Geometry: final body of the model. Coordinates: model frame, mm. Face numbers are marked on the shaded views. A direction names the side the tool comes from. Give positions to 0.01 mm unless a question says otherwise; leave off trailing zeros. Loops run counter-clockwise (first coordinate to the right, second up) from the corner with the lowest first, then second, coordinate; pieces in that order, holes last.
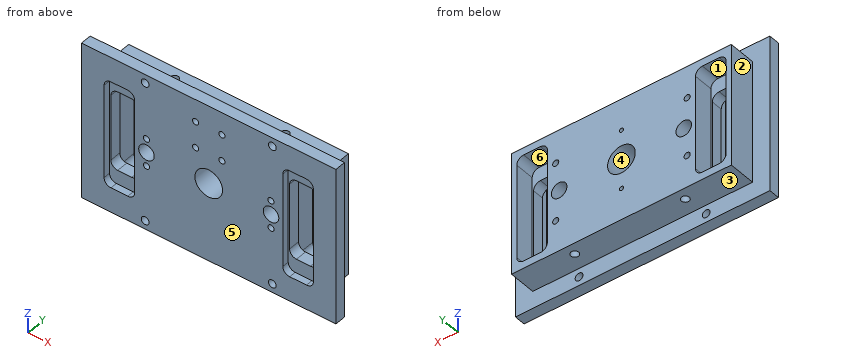
```python
from build123d import *

# Parameters (mm, degrees)
MAIN_SKETCH_W                         = 73.5
MAIN_SKETCH_H                         = 45.5
MAIN_SKETCH_W_2                       = 8.85
MAIN_SKETCH_H_2                       = 31.2
MAIN_SKETCH_R                         = 2.2479
LIP_DEPTH                             = 3.175
MOUNTING_BASE_OUTLINE_W               = 63.5
MOUNTING_BASE_OUTLINE_H               = 35.5
MOUNTING_BASE_OUTLINE_R               = 2.2479
MOUNTING_BASE_OUTLINE_R_2             = 4
MOUNTING_BASE_DEPTH                   = 11
HEATER_CART_4_40_TAPS_D               = 2.2606
HEATER_CART_4_40_TAPS_DEPTH           = 8.255
HEATER_CART_4_40_TAPS_TIP             = 0.679152758
HEATER_CART_4_40_TAPS_ON_FACE_2_D     = 2.2606
HEATER_CART_4_40_TAPS_ON_FACE_2_DEPTH = 8.255
HEATER_CART_4_40_TAPS_ON_FACE_2_TIP   = 0.679152758
MAIN_SKETCH_12_W                      = 8.85
MAIN_SKETCH_12_H                      = 31.2
MAIN_SKETCH_12_R                      = 0.285
BOTTOM_SQUARE_CUTOUT_DEPTH            = 2
SQUARE_MICRO_D_CUTOUT_START           = 5.3
SQUARE_MICRO_D_CUTOUT_OUTLINE_W       = 8.85
SQUARE_MICRO_D_CUTOUT_OUTLINE_H       = 31.2
SQUARE_MICRO_D_CUTOUT_OUTLINE_R       = 0.285
SQUARE_MICRO_D_CUTOUT_DEPTH           = 5.7
SKETCH15_W                            = 8.067488146
SKETCH15_H                            = 23.070933647
CUT_EXTRUDE1_DEPTH                    = 11
INTERNAL_CORNER_CUTOUTS_FILLET_R      = 2
CHIP_CLAMP_0_80_TAPS_AT_2_COUNT       = 2
CHIP_CLAMP_0_80_TAPS_AT_2_PITCH       = 17.1232
CHIP_CLAMP_0_80_TAPS_AT_3_COUNT       = 2
CHIP_CLAMP_0_80_TAPS_AT_3_PITCH       = 17.1232
F_2_56_CLOSE_CLEAR_43_0_089_D         = 2.2606
PCB_2_56_TAPS_D                       = 1.778
PCB_2_56_TAPS_DEPTH                   = 5.734
PCB_2_56_TAPS_TIP                     = 0.53416509
BOTTOM_COVER_2_56_TAPS_D              = 1.778
BOTTOM_COVER_2_56_TAPS_DEPTH          = 5.734
BOTTOM_COVER_2_56_TAPS_TIP            = 0.53416509
F_2_56_TAPPED_HOLE1_D                 = 1.778
F_2_56_TAPPED_HOLE1_DEPTH             = 5.734
F_2_56_TAPPED_HOLE1_TIP               = 0.53416509


# Read off the part's stored shape, not the designer's step: Mounting_Base, Square_Micro_D_Cutout
with BuildPart() as part:
    # Main_Sketch → Lip (new body)
    with BuildSketch(Plane(origin=(0, 0, 0), x_dir=(1, 0, 0), z_dir=(0, 1, 0))):
        with Locations((36.75, -22.75)):
            Rectangle(MAIN_SKETCH_W, MAIN_SKETCH_H)
        with Locations((10.925, -22.749999985)):
            Rectangle(MAIN_SKETCH_W_2, MAIN_SKETCH_H_2, mode=Mode.SUBTRACT)
        with Locations(Location((18.75, -22.75, 0), (0, 0, 270))):
            Circle(MAIN_SKETCH_R, mode=Mode.SUBTRACT)
        with BuildLine():
            ThreePointArc((31.675, -20.175), (29.907233047, -15.907233047), (34.175, -17.675))
            Line((34.175, -17.675), (39.325, -17.675))
            ThreePointArc((39.325, -17.675), (43.592766953, -15.907233047), (41.825, -20.175))
            Line((41.825, -20.175), (41.825, -25.325))
            ThreePointArc((41.825, -25.325), (43.592766953, -29.592766953), (39.325, -27.825))
            Line((39.325, -27.825), (34.175, -27.825))
            ThreePointArc((34.175, -27.825), (29.907233047, -29.592766953), (31.675, -25.325))
            Line((31.675, -25.325), (31.675, -20.175))
        make_face(mode=Mode.SUBTRACT)
        with Locations(Location((54.75, -22.75, 0), (0, 0, 270))):
            Circle(MAIN_SKETCH_R, mode=Mode.SUBTRACT)
    extrude(amount=LIP_DEPTH)

    # Mounting_Base outline → Mounting_Base (add)
    with BuildSketch(Plane(origin=(0, 0, 0), x_dir=(1, 0, 0), z_dir=(0, 1, 0))):
        with Locations((36.75, -22.75)):
            Rectangle(MOUNTING_BASE_OUTLINE_W, MOUNTING_BASE_OUTLINE_H)
        with Locations((18.75, -22.75)):
            Circle(MOUNTING_BASE_OUTLINE_R, mode=Mode.SUBTRACT)
        with Locations((54.75, -22.75)):
            Circle(MOUNTING_BASE_OUTLINE_R, mode=Mode.SUBTRACT)
        with Locations((36.75, -22.75)):
            Circle(MOUNTING_BASE_OUTLINE_R_2, mode=Mode.SUBTRACT)
    extrude(amount=MOUNTING_BASE_DEPTH)

    # Heater_Cart_#4-40_Taps
    with Locations(Plane(origin=(52.725, 7.825, 5), x_dir=(-1, 0, 0), z_dir=(0, 0, -1))):
        with Locations((0, 0), (31.95, 0)):
            Hole(HEATER_CART_4_40_TAPS_D / 2, depth=HEATER_CART_4_40_TAPS_DEPTH)
            with Locations((0, 0, -(HEATER_CART_4_40_TAPS_DEPTH + HEATER_CART_4_40_TAPS_TIP / 2))):  # 118° drill point
                Cone(0, HEATER_CART_4_40_TAPS_D / 2, HEATER_CART_4_40_TAPS_TIP, mode=Mode.SUBTRACT)

    # Heater_Cart_#4-40_Taps on face 2
    with Locations(Plane(origin=(20.775, 7.825, 40.5), x_dir=(1, 0, 0), z_dir=(0, 0, 1))):
        with Locations((0, 0), (31.95, 0)):
            Hole(HEATER_CART_4_40_TAPS_ON_FACE_2_D / 2, depth=HEATER_CART_4_40_TAPS_ON_FACE_2_DEPTH)
            with Locations((0, 0, -(HEATER_CART_4_40_TAPS_ON_FACE_2_DEPTH + HEATER_CART_4_40_TAPS_ON_FACE_2_TIP / 2))):  # 118° drill point
                Cone(0, HEATER_CART_4_40_TAPS_ON_FACE_2_D / 2, HEATER_CART_4_40_TAPS_ON_FACE_2_TIP, mode=Mode.SUBTRACT)

    # Main_Sketch<12> → Bottom_square_cutout (cut)
    # profile 1 of 2: a face of its own
    with BuildSketch(Plane(origin=(0, 0, 0), x_dir=(1, 0, 0), z_dir=(0, 1, 0))):
        with Locations((10.925, -22.749999985)):
            Rectangle(MAIN_SKETCH_12_W, MAIN_SKETCH_12_H)
        with BuildLine():
            ThreePointArc((10.385689992, -35.285466808), (9.155254643, -35.471894814), (7.986136174, -35.045410869))
            ThreePointArc((7.986136174, -35.045410869), (7.18175843, -34.143309058), (6.891255927, -32.970099985))
            Line((6.891255927, -32.970099985), (6.891255927, -12.529899985))
            ThreePointArc((6.891255927, -12.529899985), (7.18175845, -11.356690961), (7.986136174, -10.454589189))
            ThreePointArc((7.986136174, -10.454589189), (9.155254643, -10.028105244), (10.385689992, -10.21453325))
            Line((10.385689992, -10.21453325), (13.424612074, -11.500982853))
            ThreePointArc((13.424612074, -11.500982853), (14.540409069, -12.427601581), (14.958744073, -13.816349588))
            Line((14.958744073, -13.816349588), (14.958744073, -31.683650456))
            ThreePointArc((14.958744073, -31.683650456), (14.540409073, -33.072398471), (13.424612074, -33.999017205))
            Line((13.424612074, -33.999017205), (10.385689992, -35.285466808))
        make_face(mode=Mode.SUBTRACT)
    # profile 2 of 2: a face of its own
    with BuildSketch(Plane(origin=(0, 0, 0), x_dir=(1, 0, 0), z_dir=(0, 1, 0))):
        with BuildLine():
            ThreePointArc((7.986136174, -35.045410869), (7.18175843, -34.143309058), (6.891255927, -32.970099985))
            Line((6.891255927, -32.970099985), (6.891255927, -12.529899985))
            ThreePointArc((6.891255927, -12.529899985), (7.18175845, -11.356690961), (7.986136174, -10.454589189))
            ThreePointArc((7.986136174, -10.454589189), (9.155254643, -10.028105244), (10.385689992, -10.21453325))
            Line((10.385689992, -10.21453325), (13.424612074, -11.500982853))
            ThreePointArc((13.424612074, -11.500982853), (14.540409069, -12.427601581), (14.958744073, -13.816349588))
            Line((14.958744073, -13.816349588), (14.958744073, -31.683650456))
            ThreePointArc((14.958744073, -31.683650456), (14.540409073, -33.072398471), (13.424612074, -33.999017205))
            Line((13.424612074, -33.999017205), (10.385689992, -35.285466808))
            ThreePointArc((10.385689992, -35.285466808), (9.155254643, -35.471894814), (7.986136174, -35.045410869))
        make_face()
        with Locations(Location((10.239255927, -22.75, 0), (0, 0, 270))):
            Circle(MAIN_SKETCH_12_R, mode=Mode.SUBTRACT)
    bottom_square_cutout = extrude(amount=BOTTOM_SQUARE_CUTOUT_DEPTH, mode=Mode.SUBTRACT)

    # Square_Micro_D_Cutout outline → Square_Micro_D_Cutout (cut)
    with BuildSketch(Plane(origin=(0, 0, 0), x_dir=(1, 0, 0), z_dir=(0, 1, 0)).offset(SQUARE_MICRO_D_CUTOUT_START)):
        with Locations((10.925, -22.749999985)):
            Rectangle(SQUARE_MICRO_D_CUTOUT_OUTLINE_W, SQUARE_MICRO_D_CUTOUT_OUTLINE_H)
        with Locations((10.239255927, -22.75)):
            Circle(SQUARE_MICRO_D_CUTOUT_OUTLINE_R, mode=Mode.SUBTRACT)
    square_micro_d_cutout = extrude(amount=SQUARE_MICRO_D_CUTOUT_DEPTH, mode=Mode.SUBTRACT)

    # Sketch15 → Cut-Extrude1 (cut)
    with BuildSketch(Plane(origin=(0, 0, 0), x_dir=(1, 0, 0), z_dir=(0, 1, 0))):
        with Locations((10.925, -22.749999985)):
            Rectangle(SKETCH15_W, SKETCH15_H)
    cut_extrude1 = extrude(amount=CUT_EXTRUDE1_DEPTH, mode=Mode.SUBTRACT)

    # MicroD_Mirror: Bottom_square_cutout, Square_Micro_D_Cutout, Cut-Extrude1 across plane
    add(bottom_square_cutout.mirror(Plane(origin=(36.75, 0, 0), x_dir=(0, 0, 1), z_dir=(1, 0, 0))), mode=Mode.SUBTRACT)
    add(square_micro_d_cutout.mirror(Plane(origin=(36.75, 0, 0), x_dir=(0, 0, 1), z_dir=(1, 0, 0))), mode=Mode.SUBTRACT)
    add(cut_extrude1.mirror(Plane(origin=(36.75, 0, 0), x_dir=(0, 0, 1), z_dir=(1, 0, 0))), mode=Mode.SUBTRACT)

    # Internal_Corner_cutouts_fillet
    internal_corner_cutouts_fillet_edges = [part.edges().sort_by_distance(p)[0] for p in [
        (15.35, 1, 38.349999985),
        (15.35, 1, 7.149999985),
        (6.5, 1, 7.149999985),
        (6.5, 1, 38.349999985),
        (15.35, 8.15, 38.349999985),
        (6.5, 8.15, 38.349999985),
        (6.5, 8.15, 7.149999985),
        (15.35, 8.15, 7.149999985),
        (14.958744073, 3.65, 34.285466808),
        (14.958744073, 3.65, 11.214533161),
        (6.891255927, 3.65, 11.214533161),
        (6.891255927, 3.65, 34.285466808),
        (58.15, 1, 7.149999985),
        (58.15, 1, 38.349999985),
        (67, 1, 38.349999985),
        (67, 1, 7.149999985),
        (67, 8.15, 7.149999985),
        (67, 8.15, 38.349999985),
        (58.15, 8.15, 38.349999985),
        (58.15, 8.15, 7.149999985),
        (58.541255927, 3.65, 11.214533161),
        (58.541255927, 3.65, 34.285466808),
        (66.608744073, 3.65, 34.285466808),
        (66.608744073, 3.65, 11.214533161),
    ]]
    fillet(internal_corner_cutouts_fillet_edges, radius=INTERNAL_CORNER_CUTOUTS_FILLET_R)

    # Sketch3 → Chip_Clamp_#0-80 Taps (revolve, cut)
    with BuildSketch(Plane(origin=(36.75, 11, 31.3116), x_dir=(0, 0, 1), z_dir=(1, 0, 0))):
        Polygon((0, 0), (0, 4.358890611), (0.59563, 4.001), (0.59563, 0), align=None)
    chip_clamp_0_80_taps = revolve(axis=Axis((36.75, 17.35, 31.3116), (0, -1, 0)), mode=Mode.SUBTRACT)

    # Chip_Clamp_#0-80 Taps at 2: Chip_Clamp_#0-80 Taps ×2
    with Locations(*[(0, 0, -i * CHIP_CLAMP_0_80_TAPS_AT_2_PITCH) for i in range(1, CHIP_CLAMP_0_80_TAPS_AT_2_COUNT)]):
        add(chip_clamp_0_80_taps, mode=Mode.SUBTRACT)

    # Chip_Clamp_#0-80 Taps at 3: Chip_Clamp_#0-80 Taps ×2
    with Locations(*[(0, 0, -i * CHIP_CLAMP_0_80_TAPS_AT_3_PITCH) for i in range(1, CHIP_CLAMP_0_80_TAPS_AT_3_COUNT)]):
        add(chip_clamp_0_80_taps, mode=Mode.SUBTRACT)

    # 2-56_Close_Clear#43 (0.089) (through all)
    with Locations(Plane(origin=(18.375, 0, 43), x_dir=(0, 0, -1), z_dir=(0, -1, 0))):
        with Locations((0, 0), (40.5, 0), (40.5, 36.75), (0, 36.75)):
            Hole(F_2_56_CLOSE_CLEAR_43_0_089_D / 2)

    # PCB #2-56 Taps
    with Locations(Plane(origin=(17.75, 11, 14.25), x_dir=(0, 0, 1), z_dir=(0, 1, 0))):
        with Locations((0, 0), (17, 0), (0, 38), (17, 38)):
            Hole(PCB_2_56_TAPS_D / 2, depth=PCB_2_56_TAPS_DEPTH)
            with Locations((0, 0, -(PCB_2_56_TAPS_DEPTH + PCB_2_56_TAPS_TIP / 2))):  # 118° drill point
                Cone(0, PCB_2_56_TAPS_D / 2, PCB_2_56_TAPS_TIP, mode=Mode.SUBTRACT)

    # Bottom_Cover#2-56 Taps
    with Locations(Plane(origin=(54.75, 0, 18.75), x_dir=(0, 0, -1), z_dir=(0, -1, 0))):
        with Locations((0, 0), (-8, 0), (-8, -36), (0, -36)):
            Hole(BOTTOM_COVER_2_56_TAPS_D / 2, depth=BOTTOM_COVER_2_56_TAPS_DEPTH)
            with Locations((0, 0, -(BOTTOM_COVER_2_56_TAPS_DEPTH + BOTTOM_COVER_2_56_TAPS_TIP / 2))):  # 118° drill point
                Cone(0, BOTTOM_COVER_2_56_TAPS_D / 2, BOTTOM_COVER_2_56_TAPS_TIP, mode=Mode.SUBTRACT)

    # #2-56 Tapped Hole1
    with Locations(Plane(origin=(32.94, 0, 31.38), x_dir=(0, 0, -1), z_dir=(0, -1, 0))):
        with Locations((0, 0), (-7.62, 0), (-7.62, 7.62), (0, 7.62)):
            Hole(F_2_56_TAPPED_HOLE1_D / 2, depth=F_2_56_TAPPED_HOLE1_DEPTH)
            with Locations((0, 0, -(F_2_56_TAPPED_HOLE1_DEPTH + F_2_56_TAPPED_HOLE1_TIP / 2))):  # 118° drill point
                Cone(0, F_2_56_TAPPED_HOLE1_D / 2, F_2_56_TAPPED_HOLE1_TIP, mode=Mode.SUBTRACT)


solid = part.part
```
Q1. Reachability of the marked faces 5 and 6 from +Z, -Z, +X, -X, +Y, -Y: full face, straight path, thin tool, end or side. Return the list, or none.
Q2. Pin query (flat end, axial travel): pin 1 Ø2.5 at (x, z) = (55.75, 14.25) entering from -Y; pin 2 Ø1 at (x, y) = (59, 5) entering from -Z; pin 3 Ø1.7 at (y, z) = (8, 27.5) entering from +X; pin 4 Ø6 at (x, y) = (20.5, 7) entering from +Z. Return the tip coordinate at first contact, or that it passes through.
Q3. Mould query, pull axis Z, two halves, no side actions, for the marked faces 1, 2, 3 and 4. Classes: +Z half, -Z half, draft (parallel to the pull), parting line (faces both ways), or undercut.
Q4. Section query A-A, the plane x = 62. Return loops of the section in (y, z) (3 decimals), and give its area (3 significant figures).
Q5. Section query B-B, the plane x = 49.5. Return loops of the section in (y, z) (3 decimals).
Q6. Material intervals for probe 1 along X at (y, z) = (7, 22.75); probe 2 along X at (y, z) = (1.5, 39); probe 3 along X at (y, z) = (9.45, 31.25), sorted ascending.
Q7. Section query C-C, the plane y = 1.25. State how many separate pieces and enclosed holes the cut face has, and give its area (3 significant figures).
Resolved:
1. face 5: +Z, -Z, +X, -X, -Y
1. face 6: +Y
2. pin 1: stops at y = 0
2. pin 2: stops at z = 5
2. pin 3: stops at x = 68.5
2. pin 4: stops at z = 40.5
3. face 1: undercut
3. face 2: draft
3. face 3: -Z half
3. face 4: undercut
4. outline: (0, 0) - (3.175, 0) - (3.175, 5) - (11, 5) - (11, 7.15) - (5.3, 7.15) - (5.3, 11.215) - (2, 11.215) - (2, 7.15) - (0, 7.15) - close; (0, 38.35) - (2, 38.35) - (2, 34.285) - (5.3, 34.285) - (5.3, 38.35) - (11, 38.35) - (11, 40.5) - (3.175, 40.5) - (3.175, 45.5) - (0, 45.5) - close
4. area: 106 mm2
5. outline: (0, 0) - (3.175, 0) - (3.175, 5) - (11, 5) - (11, 40.5) - (3.175, 40.5) - (3.175, 45.5) - (0, 45.5) - close
6. probe 1: x = 5 to 6.5, 15.35 to 16.5, 21 to 32.75, 40.75 to 52.5, 57 to 58.15, 67 to 68.5
6. probe 2: x = 0 to 32.05, 33.83 to 39.67, 41.45 to 73.5
6. probe 3: x = 5 to 6.5, 15.35 to 16.86, 18.64 to 36.16, 37.34 to 54.86, 56.64 to 58.15, 67 to 68.5
7. separate pieces: 1
7. enclosed holes: 17
7. area: 2,680 mm2
